```python
from build123d import *

# Parameters (mm, degrees)
CROQUIS1_W              = 390
CROQUIS1_H              = 230
SALIENTE_EXTRUIR1_DEPTH = 5.5
CROQUIS2_W              = 30
CROQUIS2_H              = 30
CORTAR_EXTRUIR1_DEPTH   = 5.5
CROQUIS3_W              = 38.5
CROQUIS3_H              = 30
CORTAR_EXTRUIR2_DEPTH   = 5.5
CROQUIS4_W              = 30
CROQUIS4_H              = 38.5
CORTAR_EXTRUIR3_DEPTH   = 5.5
CROQUIS5_W              = 30
CROQUIS5_H              = 38.5
CORTAR_EXTRUIR4_DEPTH   = 5.5
CROQUIS6_W              = 68.5
CROQUIS6_H              = 11
CORTAR_EXTRUIR5_DEPTH   = 5.5
CROQUIS7_W              = 68.5
CROQUIS7_H              = 11
CORTAR_EXTRUIR6_DEPTH   = 5.5
CROQUIS8_W              = 30
CROQUIS8_H              = 30
CORTAR_EXTRUIR7_DEPTH   = 5.5
CROQUIS9_W              = 30
CROQUIS9_H              = 38.5
CORTAR_EXTRUIR8_DEPTH   = 5.5
CROQUIS10_R             = 4.25
CORTAR_EXTRUIR9_DEPTH   = 5.5
CORTAR_EXTRUIR10_DEPTH  = 5.5
CORTAR_EXTRUIR11_DEPTH  = 5.5
CROQUIS13_W             = 5.857775835
CROQUIS13_H             = 5.857775835
CORTAR_EXTRUIR12_DEPTH  = 5.5
CORTAR_EXTRUIR13_DEPTH  = 5.5
CORTAR_EXTRUIR14_DEPTH  = 5.5
CROQUIS16_W             = 5
CROQUIS16_H             = 5
CORTAR_EXTRUIR15_DEPTH  = 5.5
CROQUIS17_R             = 4.5
CORTAR_EXTRUIR16_DEPTH  = 10
CORTAR_EXTRUIR17_DEPTH  = 10
CROQUIS19_R             = 1.5
CORTAR_EXTRUIR19_DEPTH  = 10
CROQUIS20_W             = 30
CROQUIS20_H             = 38.5
CORTAR_EXTRUIR20_DEPTH  = 10
CROQUIS21_R             = 4.25
CORTAR_EXTRUIR21_DEPTH  = 10
CROQUIS22_R             = 4.25
SALIENTE_EXTRUIR2_DEPTH = 10
CROQUIS23_W             = 8.291515613
CROQUIS23_H             = 2.906343814
CROQUIS23_W_2           = 14.865311346
CROQUIS23_H_2           = 4.543446559
CORTAR_EXTRUIR22_DEPTH  = 10
CROQUIS24_W             = 38.5
CROQUIS24_H             = 11
CORTAR_EXTRUIR23_DEPTH  = 10
CROQUIS25_W             = 38.5
CROQUIS25_H             = 11
CORTAR_EXTRUIR24_DEPTH  = 10
CROQUIS26_W             = 403.89450598
CROQUIS26_H             = 21.330606429
CORTAR_EXTRUIR25_DEPTH  = 10


with BuildPart() as part:
    # Croquis1 → Saliente-Extruir1 (new body)
    with BuildSketch(Plane(origin=(0, 0, 0), x_dir=(1, 0, 0), z_dir=(0, 1, 0))):
        Rectangle(CROQUIS1_W, CROQUIS1_H)
    extrude(amount=SALIENTE_EXTRUIR1_DEPTH)

    # Croquis2 → Cortar-Extruir1 (cut)
    with BuildSketch(Plane(origin=(0, 5.5, 0), x_dir=(1, 0, 0), z_dir=(0, 1, 0))):
        with Locations((-180, 100)):
            Rectangle(CROQUIS2_W, CROQUIS2_H)
        with Locations((180, 100)):
            Rectangle(CROQUIS2_W, CROQUIS2_H)
    extrude(amount=-CORTAR_EXTRUIR1_DEPTH, mode=Mode.SUBTRACT)

    # Croquis3 → Cortar-Extruir2 (cut)
    with BuildSketch(Plane(origin=(0, 5.5, 0), x_dir=(1, 0, 0), z_dir=(0, 1, 0))):
        with Locations((-145.75, 100)):
            Rectangle(CROQUIS3_W, CROQUIS3_H)
        with Locations((145.75, 100)):
            Rectangle(CROQUIS3_W, CROQUIS3_H)
    extrude(amount=-CORTAR_EXTRUIR2_DEPTH, mode=Mode.SUBTRACT)

    # Croquis4 → Cortar-Extruir3 (cut)
    with BuildSketch(Plane(origin=(0, 5.5, 0), x_dir=(1, 0, 0), z_dir=(0, 1, 0))):
        with Locations((-180, 65.75)):
            Rectangle(CROQUIS4_W, CROQUIS4_H)
        with Locations((180, 65.75)):
            Rectangle(CROQUIS4_W, CROQUIS4_H)
    extrude(amount=-CORTAR_EXTRUIR3_DEPTH, mode=Mode.SUBTRACT)

    # Croquis5 → Cortar-Extruir4 (cut)
    with BuildSketch(Plane(origin=(0, 5.5, 0), x_dir=(1, 0, 0), z_dir=(0, 1, 0))):
        with Locations((-180, -95.75)):
            Rectangle(CROQUIS5_W, CROQUIS5_H)
        with Locations((180, -95.75)):
            Rectangle(CROQUIS5_W, CROQUIS5_H)
    extrude(amount=-CORTAR_EXTRUIR4_DEPTH, mode=Mode.SUBTRACT)

    # Croquis6 → Cortar-Extruir5 (cut)
    with BuildSketch(Plane(origin=(0, 5.5, 0), x_dir=(1, 0, 0), z_dir=(0, 1, 0))):
        with Locations((34.25, -109.5)):
            Rectangle(CROQUIS6_W, CROQUIS6_H)
    extrude(amount=-CORTAR_EXTRUIR5_DEPTH, mode=Mode.SUBTRACT)

    # Croquis7 → Cortar-Extruir6 (cut)
    with BuildSketch(Plane(origin=(0, 5.5, 0), x_dir=(1, 0, 0), z_dir=(0, 1, 0))):
        with Locations((-34.25, -109.5)):
            Rectangle(CROQUIS7_W, CROQUIS7_H)
    extrude(amount=-CORTAR_EXTRUIR6_DEPTH, mode=Mode.SUBTRACT)

    # Croquis8 → Cortar-Extruir7 (cut)
    with BuildSketch(Plane(origin=(0, 5.5, 0), x_dir=(1, 0, 0), z_dir=(0, 1, 0))):
        with Locations((0, -89)):
            Rectangle(CROQUIS8_W, CROQUIS8_H)
    extrude(amount=-CORTAR_EXTRUIR7_DEPTH, mode=Mode.SUBTRACT)

    # Croquis9 → Cortar-Extruir8 (cut)
    with BuildSketch(Plane(origin=(0, 5.5, 0), x_dir=(1, 0, 0), z_dir=(0, 1, 0))):
        with Locations((0, -54.75)):
            Rectangle(CROQUIS9_W, CROQUIS9_H)
    extrude(amount=-CORTAR_EXTRUIR8_DEPTH, mode=Mode.SUBTRACT)

    # Croquis10 → Cortar-Extruir9 (cut)
    with BuildSketch(Plane(origin=(0, 5.5, 0), x_dir=(1, 0, 0), z_dir=(0, 1, 0))):
        with Locations(Location((-111.5, 100, 0), (0, 0, 270))):
            Circle(CROQUIS10_R)
        with Locations(Location((111.5, 100, 0), (0, 0, 270))):
            Circle(CROQUIS10_R)
        with Locations(Location((-180, 31.5, 0), (0, 0, 270))):
            Circle(CROQUIS10_R)
        with Locations(Location((-180, -61.5, 0), (0, 0, 270))):
            Circle(CROQUIS10_R)
        with Locations(Location((180, 31.5, 0), (0, 0, 270))):
            Circle(CROQUIS10_R)
        with Locations(Location((180, -61.5, 0), (0, 0, 270))):
            Circle(CROQUIS10_R)
    extrude(amount=-CORTAR_EXTRUIR9_DEPTH, mode=Mode.SUBTRACT)

    # Croquis11 → Cortar-Extruir10 (cut)
    with BuildSketch(Plane(origin=(0, 5.5, 0), x_dir=(1, 0, 0), z_dir=(0, 1, 0))):
        Polygon((126.5, 85), (127.25, 85), (126.5, 84.25), (125.75, 85), (126.5, 85.75), align=None)
    extrude(amount=-CORTAR_EXTRUIR10_DEPTH, mode=Mode.SUBTRACT)

    # Croquis12 → Cortar-Extruir11 (cut)
    with BuildSketch(Plane(origin=(0, 5.5, 0), x_dir=(1, 0, 0), z_dir=(0, 1, 0))):
        Polygon((125.75, 85), (125.573223305, 85.176776695), (126.5, 86.103553391), (127.603553391, 85), (126.676776695, 84.073223305), align=None)
    extrude(amount=-CORTAR_EXTRUIR11_DEPTH, mode=Mode.SUBTRACT)

    # Croquis13 → Cortar-Extruir12 (cut)
    with BuildSketch(Plane(origin=(0, 5.5, 0), x_dir=(1, 0, 0), z_dir=(0, 1, 0))):
        with Locations((123.571112083, 82.071112083)):
            Rectangle(CROQUIS13_W, CROQUIS13_H)
    extrude(amount=-CORTAR_EXTRUIR12_DEPTH, mode=Mode.SUBTRACT)

    # Croquis14 → Cortar-Extruir13 (cut)
    with BuildSketch(Plane(origin=(0, 5.5, 0), x_dir=(1, 0, 0), z_dir=(0, 1, 0))):
        Polygon((125.770357071, 85.373910462), (126.873910462, 84.270357071), (125.903673954, 83.300120564), (124.800120564, 84.403673954), align=None)
    extrude(amount=-CORTAR_EXTRUIR13_DEPTH, mode=Mode.SUBTRACT)

    # Croquis15 → Cortar-Extruir14 (cut)
    with BuildSketch(Plane(origin=(0, 5.5, 0), x_dir=(1, 0, 0), z_dir=(0, 1, 0))):
        Polygon((-126.5, 85), (-126.5, 86.1), (-125.4, 85), (-126.5, 83.9), (-127.6, 85), align=None)
    extrude(amount=-CORTAR_EXTRUIR14_DEPTH, mode=Mode.SUBTRACT)

    # Croquis16 → Cortar-Extruir15 (cut)
    with BuildSketch(Plane(origin=(0, 5.5, 0), x_dir=(1, 0, 0), z_dir=(0, 1, 0))):
        with Locations((-124, 82.5)):
            Rectangle(CROQUIS16_W, CROQUIS16_H)
    extrude(amount=-CORTAR_EXTRUIR15_DEPTH, mode=Mode.SUBTRACT)

    # Croquis17 → Cortar-Extruir16 (cut)
    with BuildSketch(Plane(origin=(0, 5.5, 0), x_dir=(1, 0, 0), z_dir=(0, 1, 0))):
        with Locations(Location((-101.7, -89.25, 0), (0, 0, 270))):
            Circle(CROQUIS17_R)
        with Locations(Location((101.7, -89.25, 0), (0, 0, 270))):
            Circle(CROQUIS17_R)
    extrude(amount=-CORTAR_EXTRUIR16_DEPTH, mode=Mode.SUBTRACT)

    # Croquis18 → Cortar-Extruir17 (cut)
    with BuildSketch(Plane(origin=(0, 5.5, 0), x_dir=(1, 0, 0), z_dir=(0, 1, 0))):
        Polygon((-15, -104), (-53, -104), (-53, -97.5), (-21.5, -97.5), (-21.5, -66), (-15, -66), align=None)
        Polygon((15, -66), (15, -104), (53, -104), (53, -97.5), (21.5, -97.5), (21.5, -66), align=None)
    extrude(amount=-CORTAR_EXTRUIR17_DEPTH, mode=Mode.SUBTRACT)

    # Croquis19 → Cortar-Extruir19 (cut)
    with BuildSketch(Plane(origin=(0, 5.5, 0), x_dir=(1, 0, 0), z_dir=(0, 1, 0))):
        with Locations(Location((-85.5, 25.15, 0), (0, 0, 270))):
            Circle(CROQUIS19_R)
        with Locations(Location((-63.5, 25.15, 0), (0, 0, 270))):
            Circle(CROQUIS19_R)
        with Locations(Location((-11, 25.15, 0), (0, 0, 270))):
            Circle(CROQUIS19_R)
        with Locations(Location((11, 25.15, 0), (0, 0, 270))):
            Circle(CROQUIS19_R)
        with Locations(Location((63.5, 25.15, 0), (0, 0, 270))):
            Circle(CROQUIS19_R)
        with Locations(Location((85.5, 25.15, 0), (0, 0, 270))):
            Circle(CROQUIS19_R)
        with Locations(Location((-104.25, 87, 0), (0, 0, 270))):
            Circle(CROQUIS19_R)
        with Locations(Location((-104.25, 65, 0), (0, 0, 270))):
            Circle(CROQUIS19_R)
        with Locations(Location((104.25, 87, 0), (0, 0, 270))):
            Circle(CROQUIS19_R)
        with Locations(Location((104.25, 65, 0), (0, 0, 270))):
            Circle(CROQUIS19_R)
    extrude(amount=-CORTAR_EXTRUIR19_DEPTH, mode=Mode.SUBTRACT)

    # Croquis20 → Cortar-Extruir20 (cut)
    with BuildSketch(Plane(origin=(0, 5.5, 0), x_dir=(1, 0, 0), z_dir=(0, 1, 0))):
        with Locations((180, -84.75)):
            Rectangle(CROQUIS20_W, CROQUIS20_H)
        with Locations((-180, -84.75)):
            Rectangle(CROQUIS20_W, CROQUIS20_H)
    extrude(amount=-CORTAR_EXTRUIR20_DEPTH, mode=Mode.SUBTRACT)

    # Croquis21 → Cortar-Extruir21 (cut)
    with BuildSketch(Plane(origin=(0, 5.5, 0), x_dir=(1, 0, 0), z_dir=(0, 1, 0))):
        with Locations(Location((180, -50.5, 0), (0, 0, 270))):
            Circle(CROQUIS21_R)
        with Locations(Location((-180, -50.5, 0), (0, 0, 270))):
            Circle(CROQUIS21_R)
    extrude(amount=-CORTAR_EXTRUIR21_DEPTH, mode=Mode.SUBTRACT)

    # Croquis22 → Saliente-Extruir2 (add)
    with BuildSketch(Plane(origin=(0, 5.5, 0), x_dir=(1, 0, 0), z_dir=(0, 1, 0))):
        with Locations(Location((-180, -61.5, 0), (0, 0, 270))):
            Circle(CROQUIS22_R)
        with Locations(Location((180, -61.5, 0), (0, 0, 270))):
            Circle(CROQUIS22_R)
    extrude(amount=-SALIENTE_EXTRUIR2_DEPTH)

    # Croquis23 → Cortar-Extruir22 (cut)
    with BuildSketch(Plane(origin=(0, 5.5, 0), x_dir=(1, 0, 0), z_dir=(0, 1, 0))):
        with Locations((180.153411618, -66.953171907)):
            Rectangle(CROQUIS23_W, CROQUIS23_H)
        with Locations((-178.231952533, -67.77172328)):
            Rectangle(CROQUIS23_W_2, CROQUIS23_H_2)
    extrude(amount=-CORTAR_EXTRUIR22_DEPTH, mode=Mode.SUBTRACT)

    # Croquis24 → Cortar-Extruir23 (cut)
    with BuildSketch(Plane(origin=(0, 5.5, 0), x_dir=(1, 0, 0), z_dir=(0, 1, 0))):
        with Locations((145.75, -109.5)):
            Rectangle(CROQUIS24_W, CROQUIS24_H)
    extrude(amount=-CORTAR_EXTRUIR23_DEPTH, mode=Mode.SUBTRACT)

    # Croquis25 → Cortar-Extruir24 (cut)
    with BuildSketch(Plane(origin=(0, 5.5, 0), x_dir=(1, 0, 0), z_dir=(0, 1, 0))):
        with Locations((-145.75, -109.5)):
            Rectangle(CROQUIS25_W, CROQUIS25_H)
    extrude(amount=-CORTAR_EXTRUIR24_DEPTH, mode=Mode.SUBTRACT)

    # Croquis26 → Cortar-Extruir25 (cut)
    with BuildSketch(Plane.XY.offset(65.5)):
        with Locations((6.94725299, -10.665303215)):
            Rectangle(CROQUIS26_W, CROQUIS26_H)
    extrude(amount=-CORTAR_EXTRUIR25_DEPTH, mode=Mode.SUBTRACT)


solid = part.part
```
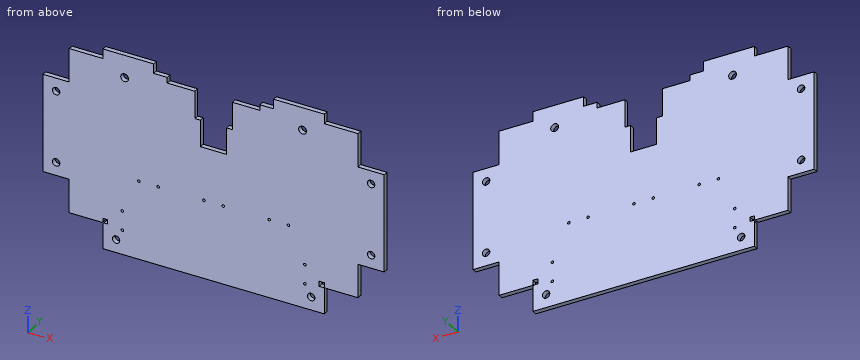
Can you work these out from the model? Positions are in its coordinate system, mm. Coordinates: 2 decimals unless noted, no trailing zeros. Write each loop counter-clockwise with the first axis right and the second up, starting at its lowest first coordinate (ties: lowest second). Pieces come first, ordered by that corner, then holes. Notation, with made-up numbers: (77.25, 38) - (110.25, 38) arc R26 ccw to (110.25, 72) - close; hole circle Ø6 at (65, -4.75). An arc over 180 degrees is marked (long way). Return JSON: item names as keys, results as strings.
Q1. If we section it at D-D (x = -42.5): Please give me the cut outline in (y, z), then the cut area to 3 significant figures.
Computed values:
{"outline": "(0, -115) - (5.5, -115) - (5.5, 97.5) - (0, 97.5) - close", "area": "1,170 mm2"}
Q2. I'm going to push flat-ended pins straight in: pin 1 Ø3 at (y, z) = (4.5, -70) entering from +X; pin 2 Ø3 at (y, z) = (4, -68.5) entering from -X; pin 3 Ø3 at (x, y) = (175, 2) entering from -Z. Where does each tip first touch, or does it pass through?
Computed values:
{"pin 1": "stops at x = 165", "pin 2": "stops at x = -165", "pin 3": "stops at z = -46.5"}
Q3. If we section it at A-A (x = 111.5): Please give me the cut outline in (y, z), then the cut area to 3 significant figures.
Computed values:
{"outline": "(0, -115) - (5.5, -115) - (5.5, -104.25) - (0, -104.25) - close; (0, -95.75) - (5.5, -95.75) - (5.5, 115) - (0, 115) - close", "area": "1,220 mm2"}
Q4. If we section it at B-B (z = -31.5): Please give me the cut outline in (x, y), then the cut area to 3 significant figures.
Computed values:
{"outline": "(-195, 0) - (-184.25, 0) - (-184.25, 5.5) - (-195, 5.5) - close; (-175.75, 0) - (175.75, 0) - (175.75, 5.5) - (-175.75, 5.5) - close; (184.25, 0) - (195, 0) - (195, 5.5) - (184.25, 5.5) - close", "area": "2,050 mm2"}
Q5. Please list where these lines run through material, in increasing order: L1, parallel to X at y = 4.45, z = -100; L2, parallel to X at y = 3.85, z = -31.5; L3, parallel to X at y = 2.25, z = 50.5. Write a range as from..to.
Computed values:
{"L1": "x = -126.5..-115.75, -107.25..107.25, 115.75..126.5", "L2": "x = -195..-184.25, -175.75..175.75, 184.25..195", "L3": "x = -195..-184.25, -175.75..-15, 15..175.75, 184.25..195"}
Q6. If we section it at C-C (y = 2.4): Count the separate pieces of the cut face and the enclosed holes in it, then the cut area to 3 significant figures.
Computed values:
{"separate pieces": "1", "enclosed holes": "18", "area": "74,400 mm2"}
